from build123d import *

# Parameters (mm, degrees)
ESQUISSE1_W             = 37
ESQUISSE1_H             = 16
BOSS_EXTRU_1_DEPTH      = 16.5
ESQUISSE3_R             = 5.5
ENL_V_MAT_EXTRU_2_DEPTH = 30.504236984
ESQUISSE14_R            = 4.5
ENL_V_MAT_EXTRU_3_DEPTH = 30.504236984
ESQUISSE15_R            = 4
ENL_V_MAT_EXTRU_4_DEPTH = 30.504236984
TROU_TARAUD_M34_REACH   = 40.668
TROU_TARAUD_M34_BORE_R  = 1.25
TROU_TARAUD_M35_REACH   = 40.668
TROU_TARAUD_M35_BORE_R  = 1.25
TROU_TARAUD_M36_REACH   = 41.444
TROU_TARAUD_M36_BORE_R  = 1.25


with BuildPart() as part:
    # Esquisse1 → Boss.-Extru.1 (new, symmetric)
    with BuildSketch(Plane(origin=(0, 0, 0), x_dir=(1, 0, 0), z_dir=(0, 1, 0))):
        Rectangle(ESQUISSE1_W, ESQUISSE1_H)
    extrude(amount=BOSS_EXTRU_1_DEPTH, both=True)

    # Esquisse3 → Enlèv. mat.-Extru.2 (cut, through all)
    with BuildSketch(Plane.XY.offset(8)):
        with Locations((11, -3.5)):
            Circle(ESQUISSE3_R)
    extrude(amount=-ENL_V_MAT_EXTRU_2_DEPTH, mode=Mode.SUBTRACT)

    # Esquisse14 → Enlèv. mat.-Extru.3 (cut, through all)
    with BuildSketch(Plane(origin=(0, 0, -8), x_dir=(-1, 0, 0), z_dir=(0, 0, -1))):
        with Locations((12, -5.8)):
            Circle(ESQUISSE14_R)
    extrude(amount=-ENL_V_MAT_EXTRU_3_DEPTH, mode=Mode.SUBTRACT)

    # Esquisse15 → Enlèv. mat.-Extru.4 (cut, through all)
    with BuildSketch(Plane(origin=(0, 0, -8), x_dir=(-1, 0, 0), z_dir=(0, 0, -1))):
        with Locations((12, 5.5)):
            Circle(ESQUISSE15_R)
    extrude(amount=-ENL_V_MAT_EXTRU_4_DEPTH, mode=Mode.SUBTRACT)

    # Trou taraudé M34 bore → Trou taraudé M34 (cut, up to next)
    with BuildSketch(Plane(origin=(0, 16.5, 0), x_dir=(1, 0, 0), z_dir=(0, 1, 0)), mode=Mode.PRIVATE) as trou_taraud_m34_sk1:
        with Locations((-12, -4.5)):
            Circle(TROU_TARAUD_M34_BORE_R)
    trou_taraud_m34_tool1 = extrude(trou_taraud_m34_sk1.sketch, amount=-TROU_TARAUD_M34_REACH, mode=Mode.PRIVATE) & part.part
    # Trou taraudé M34 bore → Trou taraudé M34 (cut, up to next)
    with BuildSketch(Plane(origin=(0, 16.5, 0), x_dir=(1, 0, 0), z_dir=(0, 1, 0)), mode=Mode.PRIVATE) as trou_taraud_m34_sk2:
        with Locations((-12, 4.5)):
            Circle(TROU_TARAUD_M34_BORE_R)
    trou_taraud_m34_tool2 = extrude(trou_taraud_m34_sk2.sketch, amount=-TROU_TARAUD_M34_REACH, mode=Mode.PRIVATE) & part.part
    add(trou_taraud_m34_tool1.solids().sort_by_distance((-12, 16.5, 4.5))[0], mode=Mode.SUBTRACT)
    add(trou_taraud_m34_tool2.solids().sort_by_distance((-12, 16.5, -4.5))[0], mode=Mode.SUBTRACT)

    # Trou taraudé M35 bore → Trou taraudé M35 (cut, up to next)
    with BuildSketch(Plane(origin=(0, -16.5, 0), x_dir=(-1, 0, 0), z_dir=(0, -1, 0)), mode=Mode.PRIVATE) as trou_taraud_m35_sk1:
        with Locations((12, -4.5)):
            Circle(TROU_TARAUD_M35_BORE_R)
    trou_taraud_m35_tool1 = extrude(trou_taraud_m35_sk1.sketch, amount=-TROU_TARAUD_M35_REACH, mode=Mode.PRIVATE) & part.part
    # Trou taraudé M35 bore → Trou taraudé M35 (cut, up to next)
    with BuildSketch(Plane(origin=(0, -16.5, 0), x_dir=(-1, 0, 0), z_dir=(0, -1, 0)), mode=Mode.PRIVATE) as trou_taraud_m35_sk2:
        with Locations((12, 4.5)):
            Circle(TROU_TARAUD_M35_BORE_R)
    trou_taraud_m35_tool2 = extrude(trou_taraud_m35_sk2.sketch, amount=-TROU_TARAUD_M35_REACH, mode=Mode.PRIVATE) & part.part
    add(trou_taraud_m35_tool1.solids().sort_by_distance((-12, -16.5, 4.5))[0], mode=Mode.SUBTRACT)
    add(trou_taraud_m35_tool2.solids().sort_by_distance((-12, -16.5, -4.5))[0], mode=Mode.SUBTRACT)

    # Trou taraudé M36 bore → Trou taraudé M36 (cut, up to next)
    with BuildSketch(Plane(origin=(-1.446004376, 16.5, -0.30351444), x_dir=(-1, 0, 0), z_dir=(0, 1, 0)), mode=Mode.PRIVATE) as trou_taraud_m36_sk1:
        with Locations((10.553995624, 0.30351444)):
            Circle(TROU_TARAUD_M36_BORE_R)
    trou_taraud_m36_tool1 = extrude(trou_taraud_m36_sk1.sketch, amount=-TROU_TARAUD_M36_REACH, mode=Mode.PRIVATE) & part.part
    add(trou_taraud_m36_tool1.solids().sort_by_distance((-12, 16.5, 0))[0], mode=Mode.SUBTRACT)


solid = part.part
The model under review builds one solid part; all positions refer to its coordinate system, in mm. A direction names the side the tool comes from. Round coordinates to 2 decimals unless told otherwise and drop trailing zeros. Write each loop counter-clockwise with the first axis right and the second up, starting at its lowest first coordinate (ties: lowest second). Pieces come first, ordered by that corner, then holes. Notation, with made-up numbers: M 19.25,12 L 41.25,12 A37 cw 41.25,51 Z; hole C 43,9 d10. An arc over 180 degrees is marked long. Use a Markdown table: item, result. Add a question column.
Q1. We need section C-C, the plane y = 5.5. State the section outline as (x, z) points.
Q2. Machinability: for faces 5 (the face through (16.08, -5.61, 0.11)), 6 (the face through (-10.75, 12.95, 0.05)), 7 (the face through (-11.73, -13.35, -3.28)), which of the approach directions +Z, -Z, +X, -X, +Y, -Y give a long, thin tool a straight path to every point of the face, cutting with its end or side? Answer none if there is none.
Q3. We need section A-A, the plane x = 11. State the section outline as (y, z) points.
Q4. We need section B-B, the plane z = -4.5. State the section outline as (x, y) points.
Q5. We need section D-D, the plane z = 0. State the section outline as (x, y) points.
Q6. Insertion check: pin 1 (2 mm diameter, centred on x = -12, z = -4.5, fed in from -Y); pin 2 (4 mm diameter, centred on x = 8.5, y = -5, fed in from -Z); pin 3 (2 mm diameter, centred on x = -12, z = -4.5, fed in from +Y). Each pin has a flat end and moves straight along its axis. Give the tip position at first contact, or say it passes through.
Q7. The part is to be moulded in two halves that separate along Y. For faces 1 (the face through (0, -16.5, 0)), 2 (the face through (-12.99, 12.95, -3.74)), 3 (the face through (-11.133, 1.595, -0.112)), 4 (the face through (-14.419, -2.006, -0.112)), say which applies: pulls with the +Y half, pulls with the -Y half, needs draft (parallel to the pull), parting line crosses it, or undercut.
Q8. To check wall thickness, follow line 1 (Z direction, x = -12, y = -15); line 2 (Z direction, x = -12, y = 12.5); line 3 (Y direction, x = -8.5, z = -1.25). State the ranges of each line that lie inside material, in increasing order.
Findings below:
| question | item | result |
|---|---|---|
| 1 | outline | M -18.5,-8 L -16,-8 L -16,8 L -18.5,8 Z; M -8,-8 L 18.5,-8 L 18.5,8 L -8,8 Z |
| 2 | face 5 | +Z, -Z |
| 2 | face 6 | +Y |
| 2 | face 7 | -Y |
| 3 | outline | M -16.5,-8 L -9,-8 L -9,8 L -16.5,8 Z; M 2,-8 L 16.5,-8 L 16.5,8 L 2,8 Z |
| 4 | outline | M -18.5,-16.5 L -13.25,-16.5 L -13.25,-10.12 A4.5 cw long -10.75,-10.12 L -10.75,-16.5 L 18.5,-16.5 L 18.5,16.5 L -10.75,16.5 L -10.75,9.3 A4 cw long -13.25,9.3 L -13.25,16.5 L -18.5,16.5 Z; hole C 11,-3.5 d11 |
| 5 | outline | M -18.5,-16.5 L 18.5,-16.5 L 18.5,16.5 L -10.75,16.5 L -10.75,9.3 A4 cw long -13.25,9.3 L -13.25,16.5 L -18.5,16.5 Z; hole C -12,-5.8 d9; hole C 11,-3.5 d11 |
| 6 | pin 1 | stops at y = -1.41 |
| 6 | pin 2 | passes through |
| 6 | pin 3 | stops at y = 1.63 |
| 7 | face 1 | pulls with the -Y half |
| 7 | face 2 | needs draft |
| 7 | face 3 | undercut |
| 7 | face 4 | undercut |
| 8 | line 1 | z = -8 to -5.75, -3.25 to 3.25, 5.75 to 8 |
| 8 | line 2 | z = -8 to -5.75, -3.25 to -1.25, 1.25 to 3.25, 5.75 to 8 |
| 8 | line 3 | y = -16.5 to -8.63, -2.97 to 3.56, 7.44 to 16.5 |
